Geometry: see drawing. Coordinates: mm, zero at the bounding-box minimum. A direction names the side the tool comes from. Coordinates: 2 decimals unless noted, no trailing zeros. Loops run counter-clockwise (first coordinate to the right, second up) from the corner with the lowest first, then second, coordinate; pieces in that order, holes last.
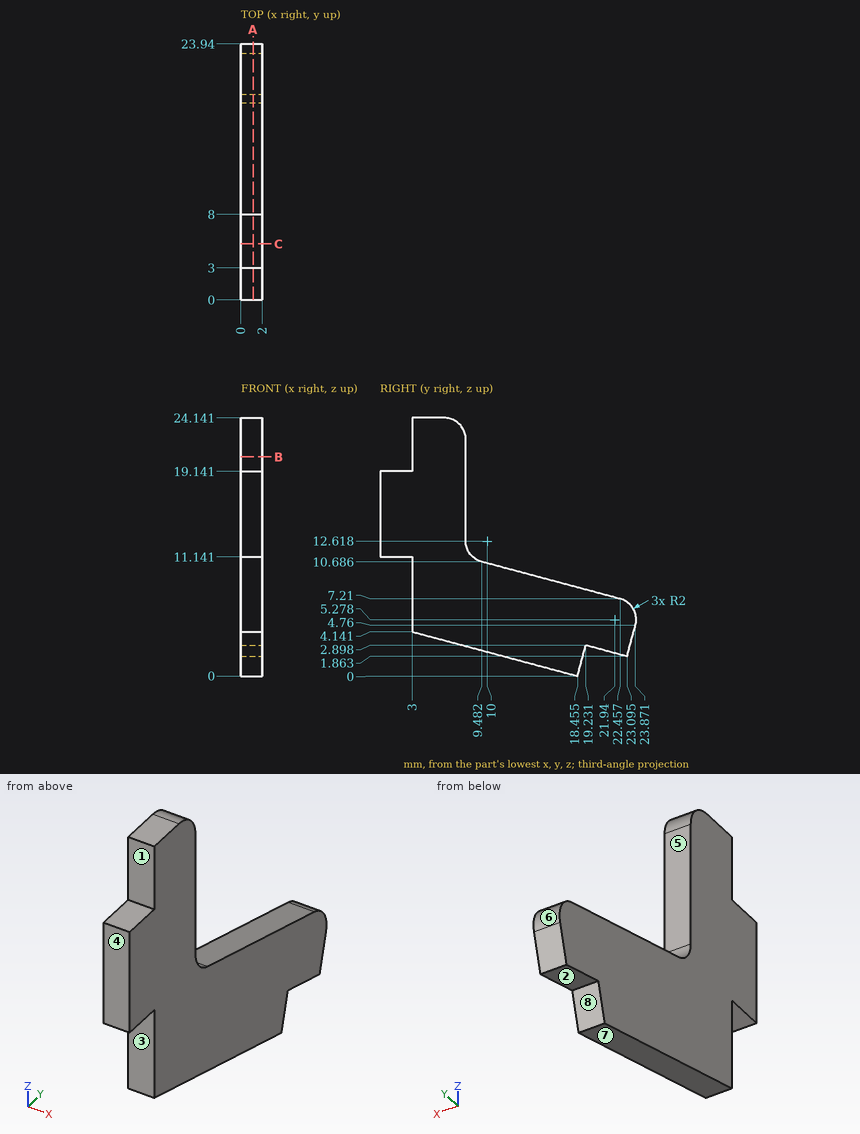
Item 1: Section query A-A (x = 1.15). Output: boundary loops of the cut face in (y, z) (1 decimal).
Result:
outline: (0, 11.1) - (3, 11.1) - (3, 4.1) - (18.5, 0) - (19.2, 2.9) - (23.1, 1.9) - (23.9, 4.8) arc R2 ccw to (22.5, 7.2) - (9.5, 10.7) arc R2 cw to (8, 12.6) - (8, 22.1) arc R2 ccw to (6, 24.1) - (3, 24.1) - (3, 19.1) - (0, 19.1) - close
Item 2: Section query B-B (z = 20.5). Output: boundary loops of the cut face in (x, y).
Result:
outline: (0, 3) - (2, 3) - (2, 8) - (0, 8) - close
Item 3: Mould query, pull axis Y, two halves, no side actions, for the marked faces 6, 7 and 8. Classes: +Y half, -Y half, draft (parallel to the pull), parting line (faces both ways), or undercut.
Result:
face 6: +Y half
face 7: -Y half
face 8: undercut
Item 4: Section query C-C (y = 5.25). Output: boundary loops of the cut face in (x, z).
Result:
outline: (0, 3.54) - (2, 3.54) - (2, 24.14) - (0, 24.14) - close
Item 5: Line query: L1, parallel to Y at x = 0.45, z = 13.75; L2, parallel to Y at x = 0.7, z = 20.5; L3, parallel to Z at x = 0.4, y = 1.5. Output: solid intervals per line, ascending.
Result:
L1: y = 0 to 8
L2: y = 3 to 8
L3: z = 11.14 to 19.14
Item 6: Reachability of the marked faces 1, 2, 3, 4 and 5 from +Z, -Z, +X, -X, +Y, -Y: full face, straight path, thin tool, end or side. Return the list, or none.
Result:
face 1: +Z, +X, -X, -Y
face 2: -Z, +X, -X
face 3: -Z, +X, -X, -Y
face 4: +Z, -Z, +X, -X, -Y
face 5: +Z, +X, -X, +Y
Item 7: Contact query for flat-ended pins moving along their axis: P1, Ø0.6, axis at x = 1, y = 2, coming from the +Z side; P2, Ø8, axis at y = 8, z = 6.5, coming from the -X side; P3, Ø0.6, axis at x = 1, z = 22, coming from the -Y side; P4, Ø0.6, axis at x = 1.5, y = 2, coming from the -Z side. Output: stop coordinate, or through.
Result:
P1: stops at z = 19.14
P2: stops at x = 0
P3: stops at y = 3
P4: stops at z = 11.14
